from build123d import *

# Parameters (mm, degrees)
PAD026_DEPTH    = 144
SKETCH044_W     = 40
SKETCH044_H     = 144
PAD027_DEPTH    = 4
SKETCH045_R     = 1.5
POCKET014_DEPTH = 5
SKETCH046_R     = 2
POCKET015_DEPTH = 4
SKETCH047_R     = 4
POCKET016_DEPTH = 7


with BuildPart() as leftfront001:
    # Sketch043 → Pad026 (new body)
    with BuildSketch(Plane.XZ):
        Polygon((0, 0), (0, 10), (7, 10), (7, 14), (-4, 14), (-4, -14), (7, -14), (7, -10), (0, -10), align=None)
    extrude(amount=PAD026_DEPTH)

    # Sketch044 (on Face4 of Pad026) → Pad027 (join)
    with BuildSketch(Plane(origin=(-4, 0, 0), x_dir=(0, 0, -1), z_dir=(-1, 0, 0))):
        with Locations((0, 72)):
            Rectangle(SKETCH044_W, SKETCH044_H)
    extrude(amount=-PAD027_DEPTH)

    # Sketch045 (on Face14 of Pad027) → Pocket014 (cut)
    with BuildSketch(Plane(origin=(-4, 0, 0), x_dir=(0, 0, -1), z_dir=(-1, 0, 0))):
        with Locations((0, 20)):
            Circle(SKETCH045_R)
        with Locations((0, 120)):
            Circle(SKETCH045_R)
    extrude(amount=-POCKET014_DEPTH, mode=Mode.SUBTRACT)

    # Sketch046 (on Face14 of Pocket014) → Pocket015 (cut)
    with BuildSketch(Plane(origin=(-4, 0, 0), x_dir=(0, 0, -1), z_dir=(-1, 0, 0))):
        with Locations((-16, 8)):
            Circle(SKETCH046_R)
        with Locations((-16, 16)):
            Circle(SKETCH046_R)
        with Locations((-16, 24)):
            Circle(SKETCH046_R)
        with Locations((-16, 32)):
            Circle(SKETCH046_R)
        with Locations((-16, 40)):
            Circle(SKETCH046_R)
        with Locations((-16, 48)):
            Circle(SKETCH046_R)
        with Locations((-16, 56)):
            Circle(SKETCH046_R)
        with Locations((-16, 64)):
            Circle(SKETCH046_R)
        with Locations((-16, 136)):
            Circle(SKETCH046_R)
        with Locations((-16, 128)):
            Circle(SKETCH046_R)
        with Locations((-16, 120)):
            Circle(SKETCH046_R)
        with Locations((-16, 112)):
            Circle(SKETCH046_R)
        with Locations((-16, 104)):
            Circle(SKETCH046_R)
        with Locations((-16, 96)):
            Circle(SKETCH046_R)
        with Locations((-16, 88)):
            Circle(SKETCH046_R)
        with Locations((-16, 80)):
            Circle(SKETCH046_R)
        with Locations((-16, 72)):
            Circle(SKETCH046_R)
        with Locations((16, 136)):
            Circle(SKETCH046_R)
        with Locations((16, 128)):
            Circle(SKETCH046_R)
        with Locations((16, 120)):
            Circle(SKETCH046_R)
        with Locations((16, 112)):
            Circle(SKETCH046_R)
        with Locations((16, 104)):
            Circle(SKETCH046_R)
        with Locations((16, 96)):
            Circle(SKETCH046_R)
        with Locations((16, 88)):
            Circle(SKETCH046_R)
        with Locations((16, 80)):
            Circle(SKETCH046_R)
        with Locations((16, 72)):
            Circle(SKETCH046_R)
        with Locations((16, 64)):
            Circle(SKETCH046_R)
        with Locations((16, 56)):
            Circle(SKETCH046_R)
        with Locations((16, 48)):
            Circle(SKETCH046_R)
        with Locations((16, 40)):
            Circle(SKETCH046_R)
        with Locations((16, 32)):
            Circle(SKETCH046_R)
        with Locations((16, 24)):
            Circle(SKETCH046_R)
        with Locations((16, 16)):
            Circle(SKETCH046_R)
        with Locations((16, 8)):
            Circle(SKETCH046_R)
    extrude(amount=-POCKET015_DEPTH, mode=Mode.SUBTRACT)

    # Sketch047 (on Face16 of Pocket014) → Pocket016 (cut)
    with BuildSketch(Plane(origin=(0, 0, 0), x_dir=(0, 0, 1), z_dir=(1, 0, 0))):
        with Locations((-16, 8)):
            Circle(SKETCH047_R)
        with Locations((-16, 16)):
            Circle(SKETCH047_R)
        with Locations((-16, 24)):
            Circle(SKETCH047_R)
        with Locations((-16, 32)):
            Circle(SKETCH047_R)
        with Locations((-16, 40)):
            Circle(SKETCH047_R)
        with Locations((-16, 48)):
            Circle(SKETCH047_R)
        with Locations((-16, 56)):
            Circle(SKETCH047_R)
        with Locations((-16, 64)):
            Circle(SKETCH047_R)
        with Locations((-16, 136)):
            Circle(SKETCH047_R)
        with Locations((-16, 128)):
            Circle(SKETCH047_R)
        with Locations((-16, 120)):
            Circle(SKETCH047_R)
        with Locations((-16, 112)):
            Circle(SKETCH047_R)
        with Locations((-16, 104)):
            Circle(SKETCH047_R)
        with Locations((-16, 96)):
            Circle(SKETCH047_R)
        with Locations((-16, 88)):
            Circle(SKETCH047_R)
        with Locations((-16, 80)):
            Circle(SKETCH047_R)
        with Locations((-16, 72)):
            Circle(SKETCH047_R)
        with Locations((16, 136)):
            Circle(SKETCH047_R)
        with Locations((16, 128)):
            Circle(SKETCH047_R)
        with Locations((16, 120)):
            Circle(SKETCH047_R)
        with Locations((16, 112)):
            Circle(SKETCH047_R)
        with Locations((16, 104)):
            Circle(SKETCH047_R)
        with Locations((16, 96)):
            Circle(SKETCH047_R)
        with Locations((16, 88)):
            Circle(SKETCH047_R)
        with Locations((16, 80)):
            Circle(SKETCH047_R)
        with Locations((16, 72)):
            Circle(SKETCH047_R)
        with Locations((16, 64)):
            Circle(SKETCH047_R)
        with Locations((16, 56)):
            Circle(SKETCH047_R)
        with Locations((16, 48)):
            Circle(SKETCH047_R)
        with Locations((16, 40)):
            Circle(SKETCH047_R)
        with Locations((16, 32)):
            Circle(SKETCH047_R)
        with Locations((16, 24)):
            Circle(SKETCH047_R)
        with Locations((16, 16)):
            Circle(SKETCH047_R)
        with Locations((16, 8)):
            Circle(SKETCH047_R)
    extrude(amount=POCKET016_DEPTH, mode=Mode.SUBTRACT)


with BuildPart() as leftfront001_1:
    # Body014 placement: moved
    add(leftfront001.part.moved(Location((-92, -59.5, 13.5))))


with BuildPart() as rightfront001:
    # Part__Mirroring003: instance of LeftFront001
    add(leftfront001_1.part.mirror(Plane(origin=(0, 0, 0), x_dir=(0, -1, 0), z_dir=(1, 0, 0))))


solid = rightfront001.part
Model file for the job. Use its own axes, mm. A direction names the side the tool comes from. Coordinates: 2 decimals unless noted, no trailing zeros. Write each loop counter-clockwise with the first axis right and the second up, starting at its lowest first coordinate (ties: lowest second). Pieces come first, ordered by that corner, then holes. Notation, with made-up numbers: (36, 81) -> (51, 81) arc R14 ccw to (51, 108) -> close; hole circle Ø11 at (-34.5, 87). An arc over 180 degrees is marked (long way). One line per item, written item: value. Start each with the question number.
1) Which spindle directions (+Z, -Z, +X, -X, +Y, -Y) get a long thin tool onto all of the face, cutting with end or side? Do faces 1 (the face through (94.028, -77.483, 29.76)), 2 (the face through (89, -201, -0.5)), 3 (the face through (88.5, -67.6, 25.5)), 4 (the face through (88.5, -67.4, 1.5)). Say none if no direction does.
2) Slice it at B-B on y = -179.5. Write the cut outline in (x, z), then the cut area to 3 significant figures.
3) Pull direction Z, two halves, no side cores. Call faces 5 (the face through (88.5, -115.6, 25.5)), 6 (the face through (88.5, -179.4, 1.5)), 7 (the face through (94.028, -193.726, 28.577)): +Z half, -Z half, draft (parallel to the pull), parting line (faces both ways), or undercut.
4) Flat gauge pins, fed straight in: pin 1 Ø4.5 at (y, z) = (-107.5, 29.5) entering from -X; pin 2 Ø0.9 at (x, y) = (88.5, -119.5) entering from -Z; pin 3 Ø0.9 at (x, y) = (89.5, -167.5) entering from +Z. Where does each tip first touch, or does it go through?
5) Probe probe 1 along Z at (x, y) = (94, -75.5); probe 2 along Y at (x, z) = (93.6, 13.5); probe 3 along Z at (x, y) = (87.5, -111). List the from-to ranges inside material, lowest first.
6) Slice it at C-C on z = 29.5. Count the separate pieces of the cut face and the enclosed holes in it, then the cut area to 3 significant figures.
7) Slice it at A-A on y = -107.5. Write the cut outline in (x, z), then the cut area to 3 significant figures.
Answers follow:
1. face 1: +X, -X
1. face 2: -Z, -X, +Y, -Y
1. face 3: +Z, -X
1. face 4: -Z, -X
2. outline: (85, 1.5) -> (92, 1.5) -> (92, -0.5) -> (96, -0.5) -> (96, 12) -> (92, 12) -> (92, 3.5) -> (85, 3.5) -> close; (85, 23.5) -> (92, 23.5) -> (92, 15) -> (96, 15) -> (96, 27.5) -> (92, 27.5) -> (92, 25.5) -> (85, 25.5) -> close; (92, -6.5) -> (96, -6.5) -> (96, -4.5) -> (92, -4.5) -> close; (92, 31.5) -> (96, 31.5) -> (96, 33.5) -> (92, 33.5) -> close
2. area: 144 mm2
3. face 5: +Z half
3. face 6: -Z half
3. face 7: undercut
4. pin 1: x = 92
4. pin 2: z = -0.5
4. pin 3: z = 27.5
5. probe 1: -6.5 to -4.5, -0.5 to 27.5, 31.5 to 33.5
5. probe 2: -203.5 to -181, -178 to -81, -78 to -59.5
5. probe 3: -0.5 to 3.5, 23.5 to 27.5
6. separate pieces: 18
6. enclosed holes: 0
6. area: 304 mm2
7. outline: (85, 1.5) -> (92, 1.5) -> (92, -0.5) -> (96, -0.5) -> (96, 27.5) -> (92, 27.5) -> (92, 25.5) -> (85, 25.5) -> (85, 23.5) -> (92, 23.5) -> (92, 3.5) -> (85, 3.5) -> close; (92, -6.5) -> (96, -6.5) -> (96, -4.5) -> (92, -4.5) -> close; (92, 31.5) -> (96, 31.5) -> (96, 33.5) -> (92, 33.5) -> close
7. area: 156 mm2
